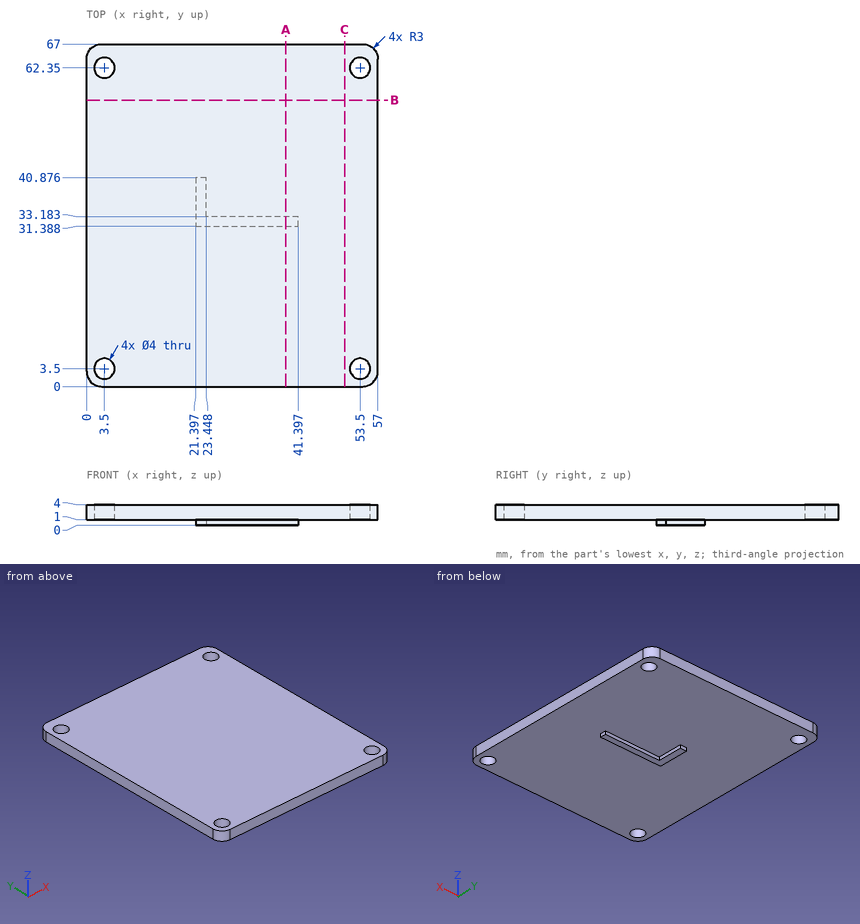
Study the drawing (mm; zero at the part's minimum x, y, z) and answer. Coordinates: 2 decimals unless noted, no trailing zeros. Write each loop counter-clockwise with the first axis right and the second up, starting at its lowest first coordinate (ties: lowest second). Pieces come first, ordered by that corner, then holes. Notation, with made-up numbers: (-15, -31) - (25, -31) arc R20 cw to (25, -17) - close; hole circle Ø4 at (20, 81). An arc over 180 degrees is marked (long way). Return JSON: item names as keys, results as strings. Group by question number.
1. A cutting plane is placed at A-A, the plane x = 39. Determine the outline of the cut face in (y, z), plus the area to 3 significant figures.
2. A cutting plane is placed at C-C, the plane x = 50.5. Determine the outline of the cut face in (y, z).
3. A cutting plane is placed at B-B, the plane y = 56. Determine the outline of the cut face in (x, z).
4. Straight lines are drawn through the part: L1, parallel to Y at x = 3.5, z = 2.65; L2, parallel to Y at x = 52.5, z = 3.5; L3, parallel to Z at x = 12.5, y = 52.5. For each, find the intervals that lie inside material, in ascending order.
5. Given pin 1 (3.5 mm diameter, centred on x = 53.5, y = 62.35, fed in from +Z); pin 2 (2 mm diameter, centred on x = 16, y = 38, fed in from -Z); pin 3 (0.8 mm diameter, centred on x = 22.5, z = 0.5, fed in from +Y), each flat-ended and moving along its own axis, determine where each tip first touches the part or whether it passes through.
Ans:
{
 "1": {"outline": "(0, 1) - (31.39, 1) - (31.39, 0) - (33.18, 0) - (33.18, 1) - (67, 1) - (67, 4) - (0, 4) - close", "area": "203 mm²"},
 "2": {"outline": "(0, 1) - (67, 1) - (67, 4) - (0, 4) - close"},
 "3": {"outline": "(0, 1) - (57, 1) - (57, 4) - (0, 4) - close"},
 "4": {"L1": "0 to 1.5, 5.5 to 60.35, 64.35 to 67", "L2": "0 to 1.77, 5.23 to 60.62, 64.08 to 67", "L3": "1 to 4"},
 "5": {"pin 1": "through", "pin 2": "z = 1", "pin 3": "y = 40.88"}
}
